The listing builds one solid part. Answer for the finished solid, in the listing's coordinates (mm). Face numbers are marked on the shaded views. A direction names the side the tool comes from. Round coordinates to 2 decimals unless told otherwise and drop trailing zeros. Write each loop counter-clockwise with the first axis right and the second up, starting at its lowest first coordinate (ties: lowest second). Pieces come first, ordered by that corner, then holes. Notation, with made-up numbers: (-32.75, 10) - (-4.75, 10) arc R12 ccw to (-4.75, 29) - close; hole circle Ø6 at (41.25, 84). An arc over 180 degrees is marked (long way). Answer as CSV lines item,"result". Start each with the question number.
Item 1: A cutting plane is placed at D-D on z = -12.5. Determine the outline of the cut face in (x, y), and give its area (3 significant figures).
Item 2: A cutting plane is placed at A-A on x = 19.5. Determine the outline of the cut face in (y, z), and give its area (3 significant figures).
Item 3: A cutting plane is placed at C-C on y = 7.75. Determine the outline of the cut face in (x, z), and give its area (3 significant figures).
Item 4: Straight lines are drawn through the part: line 1 along X through (y, z) = (0.2, -11); line 2 along X through (y, z) = (7, -11.25); line 3 along X through (y, z) = (6.2, -20). For each, find the intervals that lie inside material, in ascending order. Write a range as [from, to].
Item 5: A cutting plane is placed at B-B on z = -17.25. Determine the outline of the cut face in (x, y).
Item 6: Which of the six approach directions +Z, -Z, +X, -X, +Y, -Y give full straight-line access (tool end or side, diameter ignored) to the marked faces 5, 6, 7 and 8?
Item 7: Flat-ended cylindrical pins translate along their axes: pin 1 (3.5 mm diameter, centred on x = 19.5, z = -11, fed in from +Y); pin 2 (1.5 mm diameter, centred on y = 7, z = -12, fed in from +X); pin 3 (1.2 mm diameter, centred on x = 2, z = -2, fed in from +Y). Find the tip coordinate at first contact, or state that the pin passes through.
Item 8: For a pull along Z with two mould halves and no side action, classify the marked faces 1, 2, 3 and 4 as pulls with the +Z half, pulls with the -Z half, needs draft (parallel to the pull), parting line crosses it, or undercut.
```python
from build123d import *

# Parameters (mm, degrees)
BOSS_EXTRUDE2_DEPTH = 9
SKETCH4_W           = 5
SKETCH4_H           = 1
BOSS_EXTRUDE3_DEPTH = 5
SKETCH5_R           = 1
CUT_EXTRUDE1_DEPTH  = 5
FILLET1_R           = 1
FILLET2_R           = 1
FILLET3_R           = 3
FILLET4_R           = 3
BOSS_EXTRUDE4_DEPTH = 12
FILLET5_R           = 0.5
FILLET6_R           = 0.25
SKETCH8_R           = 3
CUT_EXTRUDE3_DEPTH  = 3
SKETCH9_R           = 0.75
CUT_EXTRUDE4_DEPTH  = 3
SKETCH10_R          = 1.5
CUT_EXTRUDE7_DEPTH  = 44.13930922
SKETCH12_R          = 1
CUT_EXTRUDE8_DEPTH  = 5
SKETCH13_W          = 1
SKETCH13_H          = 5
BOSS_EXTRUDE5_DEPTH = 2
SKETCH14_W          = 5
SKETCH14_H          = 1
BOSS_EXTRUDE6_DEPTH = 1
FILLET7_R           = 0.5
FILLET8_R           = 0.5
FILLET9_R           = 0.5
CUT_EXTRUDE9_DEPTH  = 10
SKETCH17_R          = 4.5
SKETCH17_R_2        = 1
CUT_EXTRUDE10_DEPTH = 3


with BuildPart() as part:
    # Sketch2 → Boss-Extrude2 (new body)
    with BuildSketch(Plane(origin=(0, 0, 0), x_dir=(1, 0, 0), z_dir=(0, 1, 0))):
        Polygon((0, 11), (31, 11), (31, 13.5), (31, 22), (0, 22), align=None)
        Polygon((31, 8.5), (31, 11), (0, 11), (0, 0), (31, 0), align=None)
    extrude(amount=BOSS_EXTRUDE2_DEPTH)

    # Sketch4 → Boss-Extrude3 (add)
    with BuildSketch(Plane(origin=(31, 0, 0), x_dir=(0, 0, -1), z_dir=(1, 0, 0))):
        with Locations((11, 0.5)):
            Rectangle(SKETCH4_W, SKETCH4_H)
    extrude(amount=BOSS_EXTRUDE3_DEPTH)

    # Sketch5 → Cut-Extrude1 (cut)
    with BuildSketch(Plane(origin=(0, 1, 0), x_dir=(1, 0, 0), z_dir=(0, 1, 0))):
        with Locations(Location((33.5, 11, 0), (0, 0, 270))):
            Circle(SKETCH5_R)
    extrude(amount=-CUT_EXTRUDE1_DEPTH, mode=Mode.SUBTRACT)

    # Fillet1
    fillet1_edges = [part.edges().sort_by_distance(p)[0] for p in [
        (31, 0.5, -8.5),
    ]]
    fillet(fillet1_edges, radius=FILLET1_R)

    # Fillet2
    fillet2_edges = [part.edges().sort_by_distance(p)[0] for p in [
        (31, 0.5, -13.5),
    ]]
    fillet(fillet2_edges, radius=FILLET2_R)

    # Fillet3
    fillet3_edges = [part.edges().sort_by_distance(p)[0] for p in [
        (31, 4.5, 0),
    ]]
    fillet(fillet3_edges, radius=FILLET3_R)

    # Fillet4
    fillet4_edges = [part.edges().sort_by_distance(p)[0] for p in [
        (31, 4.5, -22),
    ]]
    fillet(fillet4_edges, radius=FILLET4_R)

    # Sketch6 → Boss-Extrude4 (add)
    with BuildSketch(Plane.ZY):
        with BuildLine():
            Line((-22, 0), (-11, 0))
            Line((-11, 0), (-11, 9))
            Line((-11, 9), (-19, 9))
            ThreePointArc((-19, 9), (-21.121122912, 5.415884648), (-22, 1.344936316))
            Line((-22, 1.344936316), (-22, 0))
        make_face()
        with BuildLine():
            Line((-11, 9), (-11, 0))
            Line((-11, 0), (0, 0))
            Line((0, 0), (0, 1.344936316))
            ThreePointArc((0, 1.344936316), (-0.878877088, 5.415884648), (-3, 9))
            Line((-3, 9), (-11, 9))
        make_face()
    extrude(amount=BOSS_EXTRUDE4_DEPTH)

    # Fillet5
    fillet5_edges = [part.edges().sort_by_distance(p)[0] for p in [
        (14, 9, -22),
        (30.121320344, 9, -21.121320344),
        (31, 9, -11),
        (30.121320344, 9, -0.878679656),
        (14, 9, 0),
    ]]
    fillet(fillet5_edges, radius=FILLET5_R)

    # Fillet6
    fillet6_edges = [part.edges().sort_by_distance(p)[0] for p in [
        (36, 0.5, -13.5),
        (36, 0.5, -8.5),
    ]]
    fillet(fillet6_edges, radius=FILLET6_R)

    # Sketch8 → Cut-Extrude3 (cut)
    with BuildSketch(Plane(origin=(0, 9, 0), x_dir=(1, 0, 0), z_dir=(0, 1, 0))):
        with Locations(Location((19.5, 11, 0), (0, 0, 270))):
            Circle(SKETCH8_R)
    extrude(amount=-CUT_EXTRUDE3_DEPTH, mode=Mode.SUBTRACT)

    # Sketch9 → Cut-Extrude4 (cut)
    with BuildSketch(Plane(origin=(0, 6, 0), x_dir=(1, 0, 0), z_dir=(0, 1, 0))):
        with Locations(Location((19.5, 11, 0), (0, 0, 270))):
            Circle(SKETCH9_R)
    extrude(amount=-CUT_EXTRUDE4_DEPTH, mode=Mode.SUBTRACT)

    # Sketch10 → Cut-Extrude7 (cut, through all)
    with BuildSketch(Plane(origin=(0, 9, 0), x_dir=(1, 0, 0), z_dir=(0, 1, 0))):
        with Locations(Location((5, 19.5, 0), (0, 0, 90))):
            Circle(SKETCH10_R)
        with Locations(Location((5, 2.5, 0), (0, 0, 270))):
            Circle(SKETCH10_R)
    extrude(amount=-CUT_EXTRUDE7_DEPTH, mode=Mode.SUBTRACT)

    # Sketch12 → Cut-Extrude8 (cut)
    with BuildSketch(Plane(origin=(0, 9, 0), x_dir=(1, 0, 0), z_dir=(0, 1, 0))):
        with Locations(Location((2, 2, 0), (0, 0, 270))):
            Circle(SKETCH12_R)
        with Locations(Location((2, 20, 0), (0, 0, 270))):
            Circle(SKETCH12_R)
    extrude(amount=-CUT_EXTRUDE8_DEPTH, mode=Mode.SUBTRACT)

    # Sketch13 → Boss-Extrude5 (add)
    with BuildSketch(Plane(origin=(0, 9, 0), x_dir=(1, 0, 0), z_dir=(0, 1, 0))):
        with Locations((-7.5, 11)):
            Rectangle(SKETCH13_W, SKETCH13_H)
    extrude(amount=BOSS_EXTRUDE5_DEPTH)

    # Sketch14 → Boss-Extrude6 (add)
    with BuildSketch(Plane(origin=(-7, 0, 0), x_dir=(0, 0, -1), z_dir=(1, 0, 0))):
        with Locations((11, 10.5)):
            Rectangle(SKETCH14_W, SKETCH14_H)
    extrude(amount=BOSS_EXTRUDE6_DEPTH)

    # Fillet7
    fillet7_edges = [part.edges().sort_by_distance(p)[0] for p in [
        (-8, 11, -11),
    ]]
    fillet(fillet7_edges, radius=FILLET7_R)

    # Fillet8
    fillet8_edges = [part.edges().sort_by_distance(p)[0] for p in [
        (-8, 9, -11),
    ]]
    fillet(fillet8_edges, radius=FILLET8_R)

    # Fillet9
    fillet9_edges = [part.edges().sort_by_distance(p)[0] for p in [
        (-6, 11, -11),
    ]]
    fillet(fillet9_edges, radius=FILLET9_R)

    # Sketch16 → Cut-Extrude9 (cut)
    with BuildSketch(Plane.ZY.offset(12)):
        with BuildLine():
            Line((-18.232108037, 8.359420628), (-3.767891963, 8.359420628))
            ThreePointArc((-3.767891963, 8.359420628), (-1.809932353, 5.051006457), (-0.998661194, 1.293207997))
            Line((-0.998661194, 1.293207997), (-0.998661194, 0))
            Line((-0.998661194, 0), (-21, 0))
            Line((-21, 0), (-21.001338806, 1.293207997))
            ThreePointArc((-21.001338806, 1.293207997), (-20.190067647, 5.051006457), (-18.232108037, 8.359420628))
        make_face()
    extrude(amount=-CUT_EXTRUDE9_DEPTH, mode=Mode.SUBTRACT)

    # Sketch17 → Cut-Extrude10 (cut)
    with BuildSketch(Plane(origin=(0, 9, 0), x_dir=(1, 0, 0), z_dir=(0, 1, 0))):
        with Locations(Location((5.3, 11, 0), (0, 0, 270))):
            Circle(SKETCH17_R)
        with Locations(Location((13.3, 11, 0), (0, 0, 270))):
            Circle(SKETCH17_R_2)
    extrude(amount=-CUT_EXTRUDE10_DEPTH, mode=Mode.SUBTRACT)


solid = part.part
```
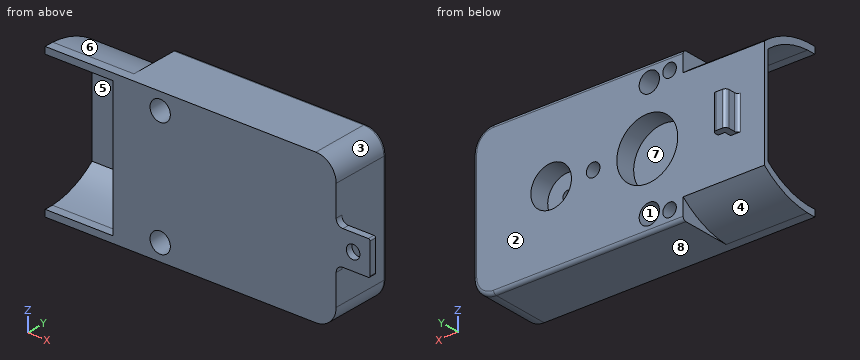
Geometry says:
1,outline,"(-12, 8.36) - (-2, 8.36) - (-2, 0) - (36, 0) - (36, 1) - (31, 1) - (31, 8.5) arc R0.5 ccw to (30.5, 9) - (22.1, 9) - (22.1, 6) - (16.9, 6) - (16.9, 9) - (9.54, 9) - (9.54, 6) - (1.06, 6) - (1.06, 9) - (-7, 9) - (-7, 10) - (-6, 10) - (-6, 10.5) arc R0.5 ccw to (-6.5, 11) - (-7.5, 11) arc R0.5 ccw to (-8, 10.5) - (-8, 9.5) arc R0.5 cw to (-8.5, 9) - (-12, 9) - close"
1,area,"270 mm^2"
2,outline,"(0, -22) - (8.5, -22) arc R0.5 ccw to (9, -21.5) - (9, -14) - (6, -14) - (6, -11.75) - (3, -11.75) - (3, -10.25) - (6, -10.25) - (6, -8) - (9, -8) - (9, -0.5) arc R0.5 ccw to (8.5, 0) - (0, 0) - close"
2,area,"175 mm^2"
3,outline,"(-12, -19.92) - (0, -19.92) - (0, -22) - (28, -22) arc R3 ccw to (31, -19) - (31, -3) arc R3 ccw to (28, 0) - (0, 0) - (0, -2.08) - (-12, -2.08) - (-12, -3.29) - (-2, -3.29) - (-2, -18.71) - (-12, -18.71) - close; hole circle Ø9 at (5.3, -11); hole circle Ø2 at (2, -20); hole circle Ø2 at (2, -2); hole circle Ø3 at (5, -19.5); hole circle Ø3 at (5, -2.5); hole circle Ø2 at (13.3, -11); hole circle Ø6 at (19.5, -11)"
3,area,"623 mm^2"
4,line 1,"x = [-2, 32.5], [34.5, 36]"
4,line 2,"x = [-2, 0.81], [9.79, 12.33], [14.27, 16.51], [22.49, 31]"
4,line 3,"x = [-12, 1], [3, 3.59], [6.41, 30.83]"
5,outline,"(-12, 8.36) - (-2, 8.36) - (-2, 0) - (31, 0) - (31, 8.5) arc R0.5 ccw to (30.5, 9) - (-12, 9) - close"
6,face 5,"-X, -Y"
6,face 6,"+Z, -X, +Y"
6,face 7,"+Y"
6,face 8,"-Z, +X, -X, +Y, -Y"
7,pin 1,"stops at y = 6"
7,pin 2,"stops at x = 31"
7,pin 3,"stops at y = 4"
8,face 1,"undercut"
8,face 2,"needs draft"
8,face 3,"pulls with the +Z half"
8,face 4,"pulls with the -Z half"
